from build123d import *

# Parameters (mm, degrees)
F1_DEPTH = 583.438
F2_DEPTH = 25.4
F3_R     = 23.8346071904
F4_DEPTH = 899.16


with BuildPart() as f1:
    # F0 (on Top) → F1 (new body)
    with BuildSketch(Plane.XY):
        Polygon((2.9511202201, -50.0551973681), (44.8246326223, -22.4718536038), (41.8735124022, 27.5833437643), (-2.9511202201, 50.0551973681), (-44.8246326223, 22.4718536038), (-41.8735124022, -27.5833437643), align=None)
    extrude(amount=F1_DEPTH)

    # F2 (add): a face of the model
    f2_faces = [f1.faces().sort_by_distance(p)[0] for p in [
        (23.8878764212, -36.263525486, 291.719),
    ]]
    extrude(f2_faces, amount=F2_DEPTH)

    # F3 (on face) → F4 (cut)
    with BuildSketch(Plane.XY.offset(583.438)):
        Circle(F3_R)
    extrude(amount=-F4_DEPTH, mode=Mode.SUBTRACT)


solid = f1.part
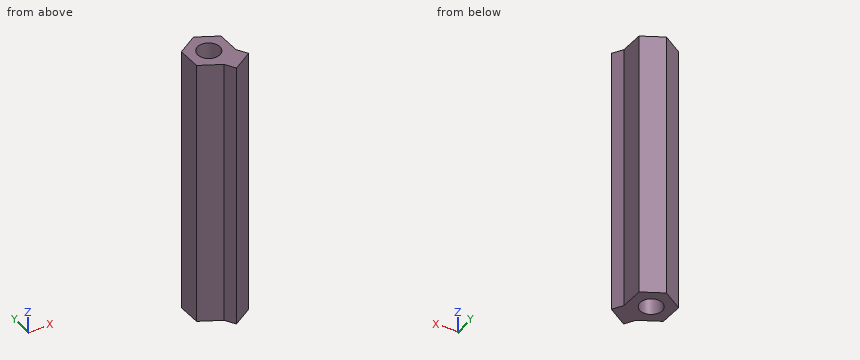
Model file for the job. Use its own axes, mm. Coordinates: 2 decimals unless noted, no trailing zeros. Write each loop counter-clockwise with the first axis right and the second up, starting at its lowest first coordinate (ties: lowest second). Pieces come first, ordered by that corner, then holes. Notation, with made-up numbers: (-25, 21) - (-12, 21) arc R18 cw to (-12, 31) - close; hole circle Ø2 at (82.25, 55.5). An arc over 180 degrees is marked (long way). Write each question's results on one line, items separated by ' | '. Start each with the question number.
1) Flat gauge pins, fed straight in: P1, Ø5, axis at x = 47.5, z = 195, coming from the -Y side; P2, Ø3, axis at y = 22, z = 476.5, coming from the +X side; P3, Ø3, axis at x = 36.5, z = 235, coming from the +Y side. Where does each tip first touch, or does it go through?
2) Cut at B-B (y = 8). Write the cut outline in (x, z).
3) Probe line 1 along Y through (x, z) = (4.5, 432); line 2 along Y through (x, z) = (0, 411); line 3 along X through (y, z) = (19, 284). List the from-to ranges inside material, lowest first. Write a range as from..to.
4) Cut at A-A (x = -13). Write the cut outline in (y, z), then the cut area to 3 significant figures.
5) Cut at D-D (y = 39). Write the cut outline in (x, z), then the cut area to 3 significant figures.
6) Cut at C-C (z = 153.5). Write the cut outline in (x, y), then the cut area to 3 significant figures.
Returned:
1) P1: y = -52.77 | P2: x = 42.29 | P3: y = 31.03
2) outline: (-43.97, 0) - (-22.45, 0) - (-22.45, 583.44) - (-43.97, 583.44) - close; (22.45, 0) - (43.03, 0) - (43.03, 583.44) - (22.45, 583.44) - close
3) line 1: -52.41..-23.41, 23.41..46.32 | line 2: -48.58..-23.83, 23.83..48.58 | line 3: -44.62..-14.39, 14.39..42.38
4) outline: (-42.06, 0) - (-19.98, 0) - (-19.98, 583.44) - (-42.06, 583.44) - close; (19.98, 0) - (43.44, 0) - (43.44, 583.44) - (19.98, 583.44) - close | area: 26,600 mm^2
5) outline: (-19.73, 0) - (19.1, 0) - (19.1, 583.44) - (-19.73, 583.44) - close | area: 22,700 mm^2
6) outline: (-44.82, 22.47) - (-41.87, -27.58) - (2.95, -50.06) - (16.92, -71.27) - (58.8, -43.68) - (44.82, -22.47) - (41.87, 27.58) - (-2.95, 50.06) - close; hole circle Ø47.67 at (0, 0) | area: 6,020 mm^2
